Input: part model. Units: mm. Frame: model coordinates. Coordinates: 2 decimals unless noted, no trailing zeros. Order: outer loops, then holes, each group sorted by start corner. A loop starts at its lowest first (then second) coordinate and runs counter-clockwise, first axis right, second up. Notation, with made-up numbers: (8.5, -11) -> (23.5, -11) arc R25 ccw to (23.5, 28) -> close; hole circle Ø2 at (38.5, 28). An arc over 180 degrees is marked (long way). One line per question, with ' | ' between items.
```python
from build123d import *

# Parameters (mm, degrees)
SKETCH1_W               = 304.8
SKETCH1_H               = 330.2
BOSS_EXTRUDE1_DEPTH     = 3.175
F_1_4_CLEARANCE_HOLE1_D = 7.14248
CUT_EXTRUDE1_REACH      = 451.383
SKETCH4_W               = 3.175
SKETCH4_H               = 69.85
SKETCH5_W               = 25.4
SKETCH5_H               = 101.6
BOSS_EXTRUDE2_DEPTH     = 3.175
F_1_4_CLEARANCE_HOLE2_D = 7.14248


with BuildPart() as part:
    # Sketch1 → Boss-Extrude1 (new body)
    with BuildSketch(Plane.XY):
        with Locations((152.4, -165.1)):
            Rectangle(SKETCH1_W, SKETCH1_H)
    extrude(amount=BOSS_EXTRUDE1_DEPTH)

    # 1/4 Clearance Hole1 (through all)
    with Locations(Plane.XY.offset(3.175)):
        with Locations((12.7, -12.7), (292.1, -12.7)):
            Hole(F_1_4_CLEARANCE_HOLE1_D / 2)

    # Sketch4 → Cut-Extrude1 (cut, up to next)
    with BuildSketch(Plane.XY.offset(3.175), mode=Mode.PRIVATE) as cut_extrude1_sk1:
        with Locations((303.2125, -130.175)):
            Rectangle(SKETCH4_W, SKETCH4_H)
    cut_extrude1_tool1 = extrude(cut_extrude1_sk1.sketch, amount=-CUT_EXTRUDE1_REACH, mode=Mode.PRIVATE) & part.part
    # Sketch4 → Cut-Extrude1 (cut, up to next)
    with BuildSketch(Plane.XY.offset(3.175), mode=Mode.PRIVATE) as cut_extrude1_sk2:
        with Locations((1.5875, -130.175)):
            Rectangle(SKETCH4_W, SKETCH4_H)
    cut_extrude1_tool2 = extrude(cut_extrude1_sk2.sketch, amount=-CUT_EXTRUDE1_REACH, mode=Mode.PRIVATE) & part.part
    add(cut_extrude1_tool1.solids().sort_by_distance((303.2125, -130.175, 3.175))[0], mode=Mode.SUBTRACT)
    add(cut_extrude1_tool2.solids().sort_by_distance((1.5875, -130.175, 3.175))[0], mode=Mode.SUBTRACT)

    # Sketch5 → Boss-Extrude2 (add)
    with BuildSketch(Plane.XY.offset(3.175)):
        with Locations((-12.7, -279.4)):
            Rectangle(SKETCH5_W, SKETCH5_H)
        with Locations((317.5, -279.4)):
            Rectangle(SKETCH5_W, SKETCH5_H)
    extrude(amount=-BOSS_EXTRUDE2_DEPTH)

    # 1/4 Clearance Hole2 (through all)
    with Locations(Plane.XY.offset(3.175)):
        with Locations((317.5, -317.5), (-12.7, -317.5)):
            Hole(F_1_4_CLEARANCE_HOLE2_D / 2)


solid = part.part
```
1. Cut plane C-C, the plane y = -116. Return loops of the section in (x, z) (3 decimals).
Recorded:
outline: (3.175, 0) -> (301.625, 0) -> (301.625, 3.175) -> (3.175, 3.175) -> close
2. Pin query (flat end, axial travel): pin 1 Ø1 at (x, z) = (323.5, 1.5) entering from +Y; pin 2 Ø1.6 at (y, z) = (-188, 1) entering from +X; pin 3 Ø1.6 at (y, z) = (-204, 1.5) entering from -X. Return the tip coordinate at first contact, or that it passes through.
Recorded:
pin 1: stops at y = -228.6 | pin 2: stops at x = 304.8 | pin 3: stops at x = 0
3. Ray query, line 1 (X direction, y = -317.5, z = 1.95); line 2 (Y direction, x = 317.5, z = 1.1); line 3 (Y direction, x = 292.1, z = 0.9). Return the intervals inside material, ascending. Write a range as [from, to].
Recorded:
line 1: x = [-25.4, -16.27], [-9.13, 313.93], [321.07, 330.2] | line 2: y = [-330.2, -321.07], [-313.93, -228.6] | line 3: y = [-330.2, -16.27], [-9.13, 0]
4. Cut plane B-B, the plane y = -21. Return loops of the section in (x, z) (3 decimals).
Recorded:
outline: (0, 0) -> (304.8, 0) -> (304.8, 3.175) -> (0, 3.175) -> close
5. Cut plane A-A, the plane z = 1.4. Return loops of the section in (x, y) (3 decimals), and give its area (3 significant figures).
Recorded:
outline: (-25.4, -330.2) -> (330.2, -330.2) -> (330.2, -228.6) -> (304.8, -228.6) -> (304.8, -165.1) -> (301.625, -165.1) -> (301.625, -95.25) -> (304.8, -95.25) -> (304.8, 0) -> (0, 0) -> (0, -95.25) -> (3.175, -95.25) -> (3.175, -165.1) -> (0, -165.1) -> (0, -228.6) -> (-25.4, -228.6) -> close; hole circle Ø7.142 at (-12.7, -317.5); hole circle Ø7.142 at (12.7, -12.7); hole circle Ø7.142 at (292.1, -12.7); hole circle Ø7.142 at (317.5, -317.5) | area: 105,000 mm^2
